Part model, mm, in its own coordinate system. A direction names the side the tool comes from. Give positions to 0.01 mm unless a question says otherwise; leave off trailing zeros. Order: outer loops, then holes, each group sorted by start corner. A loop starts at its lowest first (then second) coordinate and runs counter-clockwise, first axis right, second up. Notation, with made-up numbers: (41, 64) - (52, 64) arc R27 ccw to (52, 85) - close; hole circle Ø2 at (87, -27). An arc over 180 degrees is marked (long way). One line per item, written item: value.
```python
from build123d import *


with BuildPart() as part:
    # 扫描2: sweep along a path in 草图2
    with BuildLine(Plane(origin=(0, 0, -16.268170321), x_dir=(-1, 0, 0), z_dir=(0, 0, -1))) as sweep_2_path:
        Line((18.693353683, 0), (18.693353683, -10))
        Line((18.693353683, -10), (148.693353683, -32.922507492))
        Line((148.693353683, -32.922507492), (178.693353683, -15.601999416))
    # 草图1 → 扫描2 (sweep)
    with BuildSketch(Plane(origin=(0, 0, 0), x_dir=(1, 0, 0), z_dir=(0, 1, 0))):
        Polygon((-24.333441136, 21.518170321), (-24.333441136, 24.303170321), (-14.333441136, 24.303170321), (-14.333441136, 8.233170321), (-24.333441136, 8.233170321), (-24.333441136, 11.018170321), (-18.640334153, 11.018170321), (-18.640334153, 21.518170321), align=None)
    sweep(path=sweep_2_path.line, transition=Transition.RIGHT)


solid = part.part
```
1) Pin check, flat tips, straight feed: pin 1 (4 mm diameter, centred on y = -25.5, z = -19.5, fed in from -X); pin 2 (2 mm diameter, centred on y = -2, z = -10, fed in from -X); pin 3 (4 mm diameter, centred on y = -32, z = -16, fed in from -X); pin 4 (10 mm diameter, centred on x = -93, y = -8.5, fed in from +Z). Stop position of each tip, or through.
Outcome:
pin 1: stops at x = -173.73
pin 2: stops at x = -24.33
pin 3: stops at x = -162.48
pin 4: passes through
2) Mould opens along Z. For faces 1 (the flat face through (-163.922, -24.192, -16.342)), 2 (the flat face through (-24.333, -3, -23)), 3 (the flat face through (-97, -20, -24.303)) say: released by +Z, released by -Z, zero draft, split by the parting line, or undercut.
Outcome:
face 1: undercut
face 2: zero draft
face 3: released by -Z
3) Cut at B-B, the plane z = -16. Give the cut face in (x, y).
Outcome:
outline: (-180.87, -19.38) - (-149.5, -37.49) - (-14.33, -13.66) - (-14.33, 0) - (-18.64, 0) - (-18.64, -10.04) - (-148.7, -32.98) - (-178.72, -15.65) - close
4) Cut at C-C, the plane x = -120. Give the cut face in (y, z).
Outcome:
outline: (-32.29, -24.3) - (-22.14, -24.3) - (-22.14, -21.52) - (-27.92, -21.52) - (-27.92, -11.02) - (-22.14, -11.02) - (-22.14, -8.23) - (-32.29, -8.23) - close
5) Drill centre lines: line 1 along X through (y, z) = (-2, -17.75); line 2 along Y through (x, z) = (-31.5, -11.5); line 3 along Y through (x, z) = (-170, -22). Where is each one in solid material? Low to high. Write a range as from..to.
Outcome:
line 1: x = -18.64..-14.33
line 2: y = -16.69..-12.31
line 3: y = -25.66..-14.11
6) Which spindle directions (+Z, -Z, +X, -X, +Y, -Y) get a long thin tool onto all of the face, cutting with end or side? Do faces 4 (the flat face through (-86.9, -16.3, -22.9)), 5 (the flat face through (-24.333, -3, -10)), 6 (the flat face through (-99, -20, -21.518)). Say none if no direction does.
Outcome:
face 4: +Z, -Z, +Y
face 5: +Z, -Z, -X, +Y
face 6: +Y
7) Cut at A-A, the plane y = -29.5. Give the cut face in (x, z), then the cut area to 3 significant figures.
Outcome:
outline: (-163.34, -24.3) - (-104.18, -24.3) - (-104.18, -8.23) - (-163.34, -8.23) - close; hole (-154.73, -21.52) - (-128.98, -21.52) - (-128.98, -11.02) - (-154.73, -11.02) - close
area: 680 mm^2
